Source: CAD feature listing. Evaluate the final solid. Frame: model axes, mm. A direction names the side the tool comes from. Give positions to 0.01 mm unless a question says otherwise; leave off trailing zeros. Order: outer loops, then holes, each group sorted by start corner. A loop starts at its lowest first (then second) coordinate and runs counter-clockwise, first axis right, second up. Notation, with made-up numbers: M -7,60.25 L 7,60.25 A27 cw 7,78.25 Z; hole C -16.5,23.5 d8. An arc over 180 degrees is marked long. Return JSON: item names as keys, results as strings.
from build123d import *

# Parameters (mm, degrees)
EXTRUDE_1_DEPTH     = 4
SKETCH_2_W          = 47
SKETCH_2_H          = 26.5
SKETCH_2_W_2        = 41
SKETCH_2_H_2        = 20.5
EXTRUDE_2_DEPTH     = 43
SKETCH_3_W          = 58
SKETCH_3_H          = 30
SKETCH_3_W_2        = 41
SKETCH_3_H_2        = 20.5
EXTRUDE_3_DEPTH     = 4
SKETCH_4_W          = 43.435998006
SKETCH_4_H          = 8
CUT_EXTRUDE_1_DEPTH = 35


with BuildPart() as part:
    # 草图1 → 凸台-拉伸1 (new body)
    with BuildSketch(Plane.XY):
        with BuildLine():
            Line((-7.5, 50), (-7.5, 7.5))
            Line((-7.5, 7.5), (-50, 7.5))
            ThreePointArc((-50, 7.5), (-57.5, 0), (-50, -7.5))
            Line((-50, -7.5), (-7.5, -7.5))
            Line((-7.5, -7.5), (-7.5, -50))
            ThreePointArc((-7.5, -50), (0, -57.5), (7.5, -50))
            Line((7.5, -50), (7.5, -7.5))
            Line((7.5, -7.5), (50, -7.5))
            ThreePointArc((50, -7.5), (57.5, 0), (50, 7.5))
            Line((50, 7.5), (7.5, 7.5))
            Line((7.5, 7.5), (7.5, 50))
            ThreePointArc((7.5, 50), (0, 57.5), (-7.5, 50))
        make_face()
    extrude(amount=EXTRUDE_1_DEPTH)

    # 草图2 → 凸台-拉伸2 (add)
    with BuildSketch(Plane.XY.offset(4)):
        Rectangle(SKETCH_2_W, SKETCH_2_H)
        Rectangle(SKETCH_2_W_2, SKETCH_2_H_2, mode=Mode.SUBTRACT)
    extrude(amount=EXTRUDE_2_DEPTH)

    # 草图3 → 凸台-拉伸3 (add)
    with BuildSketch(Plane.XY.offset(47)):
        Rectangle(SKETCH_3_W, SKETCH_3_H)
        Rectangle(SKETCH_3_W_2, SKETCH_3_H_2, mode=Mode.SUBTRACT)
    extrude(amount=EXTRUDE_3_DEPTH)

    # 草图4 → 切除-拉伸1 (cut)
    with BuildSketch(Plane.XY.offset(51)):
        with Locations((17.279283878, 0)):
            Rectangle(SKETCH_4_W, SKETCH_4_H)
    extrude(amount=-CUT_EXTRUDE_1_DEPTH, mode=Mode.SUBTRACT)


solid = part.part
1. Draft query along X for faces 6 (the face through (0, 10.25, 27)), 7 (the face through (7.5, 28, 2)), 8 (the face through (0, 36, 4)), 9 (the face through (-7.5, -28, 2)). Return one class per face: pulls with the +X half, pulls with the -X half, needs draft (parallel to the pull), parting line crosses it, or undercut.
Evaluation:
{"face 6": "undercut", "face 7": "pulls with the +X half", "face 8": "needs draft", "face 9": "pulls with the -X half"}
2. Section query B-B (z = 44). Return loops of the section in (x, y).
Evaluation:
{"outline": "M -23.5,-13.25 L 23.5,-13.25 L 23.5,-4 L 20.5,-4 L 20.5,-10.25 L -20.5,-10.25 L -20.5,10.25 L 20.5,10.25 L 20.5,4 L 23.5,4 L 23.5,13.25 L -23.5,13.25 Z"}
3. Set-up query: faces 1 (the face through (-23.5, 0, 25)), 2 (the face through (0, -13.25, 25)), 3 (the face through (22, 0, 16)), 4 (the face through (20.5, -5, 27)), 5 (the face through (23.5, 6, 25)). Return all of +Z, -Z, +X, -X, +Y, -Y with unobstructed straight access to the full face (end or side cutting, diameter ignored); none if empty.
Evaluation:
{"face 1": "-X, +Y, -Y", "face 2": "+X, -X, -Y", "face 3": "+Z, +X", "face 4": "+Z", "face 5": "+X, +Y, -Y"}
4. Section query C-C (x = 0). Return loops of the section in (y, z).
Evaluation:
{"outline": "M -57.5,0 L 57.5,0 L 57.5,4 L 13.25,4 L 13.25,47 L 15,47 L 15,51 L 10.25,51 L 10.25,4 L -10.25,4 L -10.25,51 L -15,51 L -15,47 L -13.25,47 L -13.25,4 L -57.5,4 Z"}
5. Section query A-A (x = 18). Return loops of the section in (y, z), then the cut area to 3 significant figures.
Evaluation:
{"outline": "M -15,47 L -13.25,47 L -13.25,4 L -10.25,4 L -10.25,51 L -15,51 Z; M -7.5,0 L 7.5,0 L 7.5,4 L -7.5,4 Z; M 10.25,4 L 13.25,4 L 13.25,47 L 15,47 L 15,51 L 10.25,51 Z", "area": "356 mm^2"}
6. First-contact query: pin 1 (1.2 mm diameter, centred on y = 27, z = 3, fed in from +X); pin 2 (4.5 mm diameter, centred on x = 36, y = 2, fed in from +Z); pin 3 (2 mm diameter, centred on y = 25, z = 1.5, fed in from -X). Flat tips, straight axial feed; report the tip coordinate or a pass-through.
Evaluation:
{"pin 1": "stops at x = 7.5", "pin 2": "stops at z = 4", "pin 3": "stops at x = -7.5"}
7. Ray query, probe 1 along Y at (x, z) = (-15.5, 33); probe 2 along X at (y, z) = (0, 7); probe 3 along Z at (x, y) = (-3.5, -1). Return the intervals inside material, ascending.
Evaluation:
{"probe 1": "y = -13.25 to -10.25, 10.25 to 13.25", "probe 2": "x = -23.5 to -20.5, 20.5 to 23.5", "probe 3": "z = 0 to 4"}
8. Section query D-D (y = 0). Return loops of the section in (x, z).
Evaluation:
{"outline": "M -57.5,0 L 57.5,0 L 57.5,4 L 23.5,4 L 23.5,16 L 20.5,16 L 20.5,4 L -20.5,4 L -20.5,51 L -29,51 L -29,47 L -23.5,47 L -23.5,4 L -57.5,4 Z"}
